Input: dimensioned drawing with shaded views. Units: mm. Origin: part minimum x, y, z. Round coordinates to 2 decimals unless told otherwise and drop trailing zeros. Loops run counter-clockwise (first coordinate to the right, second up) from the corner with the lowest first, then second, coordinate; pieces in that order, holes last. Notation, with made-up numbers: (-33, -18.75) - (23, -18.75) arc R24 cw to (23, 18.25) - close; hole circle Ø11 at (47.25, 86). An arc over 180 degrees is marked (long way). Answer as a JSON object with one key per item and string values. Group by question number.
Item 1: Section D-D (x = 8.25). Return the cut outline in (y, z).
Item 2: Section C-C (x = 17.5). Return the cut outline in (y, z), plus the area to 3 significant figures.
Item 3: Section A-A (z = 12). Return the cut outline in (x, y).
Item 4: First-contact query: pin 1 (6.5 mm diameter, centred on x = 10.5, y = 15, fed in from -Z). Flat tip, straight axial feed; report the tip coordinate or a pass-through.
Item 5: Draft query along Z for the marked faces 1, 2 and 3. Return one class per face: released by +Z, released by -Z, zero draft, split by the parting line, or undercut.
Item 6: Line query: line 1 (Y direction, x = 10.5, z = 10.25); line 2 (Y direction, x = 13, z = 16.75); line 3 (Y direction, x = 10.5, z = 13). Output: solid intervals per line, ascending.
Item 7: Section B-B (y = 15). Return the cut outline in (x, z), plus the area to 3 significant figures.
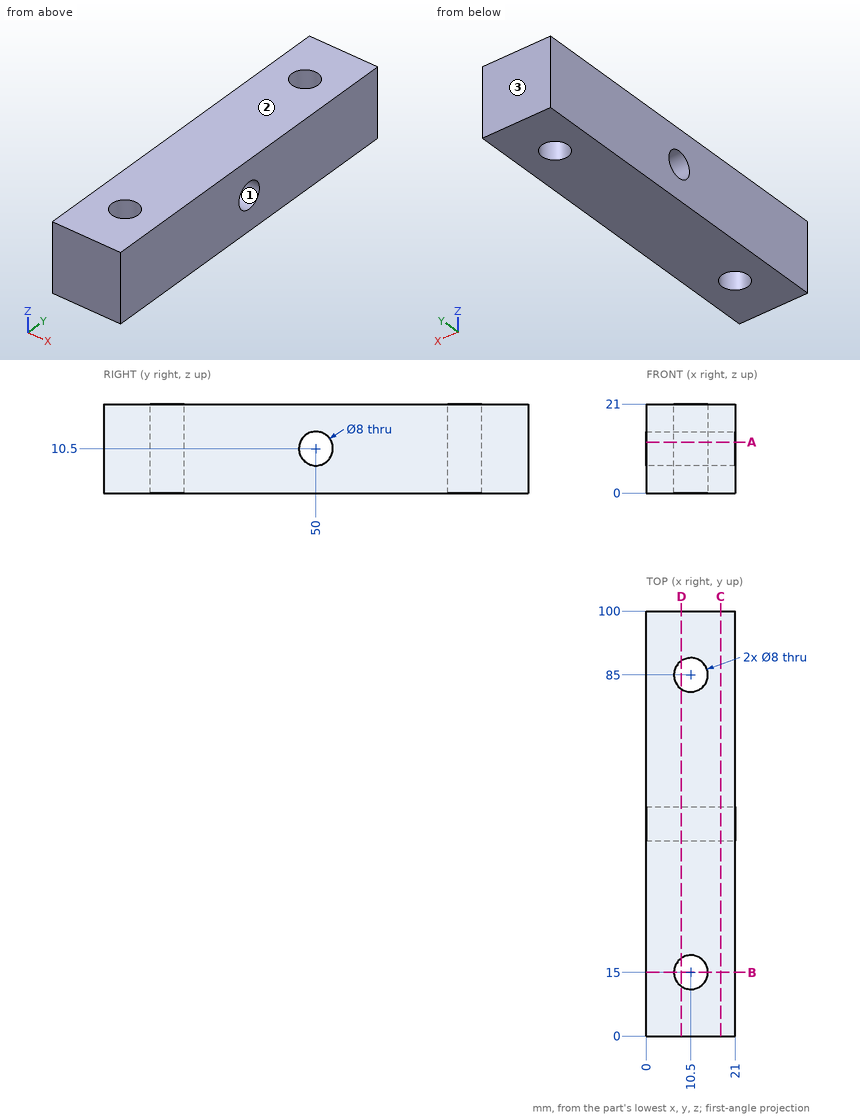
Values:
{
 "1": {"outline": "(0, 0) - (11.69, 0) - (11.69, 21) - (0, 21) - close; (18.31, 0) - (81.69, 0) - (81.69, 21) - (18.31, 21) - close; (88.31, 0) - (100, 0) - (100, 21) - (88.31, 21) - close; hole circle Ø8 at (50, 10.5)"},
 "2": {"outline": "(0, 0) - (100, 0) - (100, 21) - (0, 21) - close; hole circle Ø8 at (50, 10.5)", "area": "2,050 mm^2"},
 "3": {"outline": "(0, 0) - (21, 0) - (21, 46.29) - (0, 46.29) - close; (0, 53.71) - (21, 53.71) - (21, 100) - (0, 100) - close; hole circle Ø8 at (10.5, 15); hole circle Ø8 at (10.5, 85)"},
 "4": {"pin 1": "passes through"},
 "5": {"face 1": "undercut", "face 2": "released by +Z", "face 3": "zero draft"},
 "6": {"line 1": "y = 0 to 11, 19 to 46.01, 53.99 to 81, 89 to 100", "line 2": "y = 0 to 11.88, 18.12 to 81.88, 88.12 to 100", "line 3": "y = 0 to 11, 19 to 46.88, 53.12 to 81, 89 to 100"},
 "7": {"outline": "(0, 0) - (6.5, 0) - (6.5, 21) - (0, 21) - close; (14.5, 0) - (21, 0) - (21, 21) - (14.5, 21) - close", "area": "273 mm^2"}
}
